from build123d import *

# Parameters (mm, degrees)
EXTRUDE_2_DEPTH     = 1.8
SKETCH_2_R          = 2
CUT_EXTRUDE_3_DEPTH = 1.8


with BuildPart() as part:
    # 草圖1 → 填料-伸長2 (new body)
    with BuildSketch(Plane.XY):
        Polygon((-40.127945462, -52.376209375), (59.872054538, -52.376209375), (82.372054538, -13.405066204), (65.051546462, -3.405066204), (42.551546462, -42.376209375), (-22.807437387, -42.376209375), (-45.307437387, -3.405066204), (-62.627945462, -13.405066204), align=None)
    extrude(amount=EXTRUDE_2_DEPTH)

    # 草圖2 → 除料-伸長3 (cut)
    with BuildSketch(Plane.XY.offset(1.8)):
        with Locations((-48.967691424, -17.065320242)):
            Circle(SKETCH_2_R)
        with Locations((68.7118005, -17.065320242)):
            Circle(SKETCH_2_R)
        with Locations((-43.967691424, -25.72557428)):
            Circle(SKETCH_2_R)
        with Locations((63.7118005, -25.72557428)):
            Circle(SKETCH_2_R)
        with Locations((-15.127945462, -47.376209375)):
            Circle(SKETCH_2_R)
        with Locations((34.872054538, -47.376209375)):
            Circle(SKETCH_2_R)
    extrude(amount=-CUT_EXTRUDE_3_DEPTH, mode=Mode.SUBTRACT)


solid = part.part
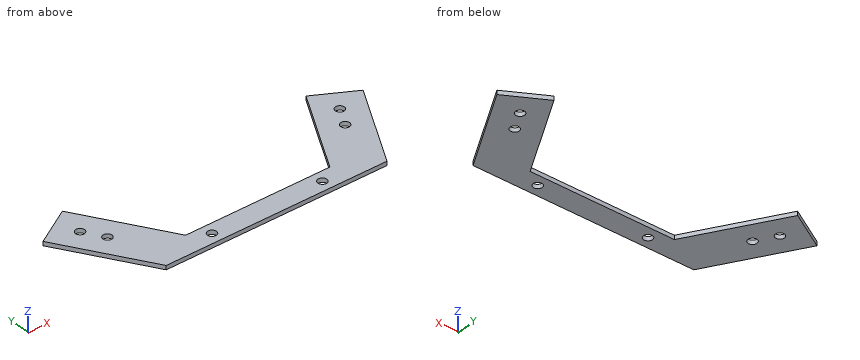
Design review of the part built by this model. Coordinates are the model's own, in mm. Round coordinates to 2 decimals unless told otherwise and drop trailing zeros. Write each loop counter-clockwise with the first axis right and the second up, starting at its lowest first coordinate (ties: lowest second). Pieces come first, ordered by that corner, then holes. Notation, with made-up numbers: (-4.5, 24) - (17.5, 24) arc R21 cw to (17.5, 54) - close; hole circle Ø8 at (60, -15.5). An arc over 180 degrees is marked (long way). Use a Markdown table: item, result. Add a question column.
1. We need section C-C (z = 1). State the section outline as (x, y) points, then the cut area to 3 significant figures.
2. Wall thickness on probe 1 along Y at (x, z) = (-15, 0.8); probe 2 along X at (y, z) = (-26.5, 1.1); probe 3 along X at (y, z) = (-47.5, 0.35): over which ranges is each line inside the solid? List them lowest first.
3. We need section D-D (x = 7.5). State the section outline as (y, z) points, then the cut area to 3 significant figures.
4. We need section A-A (y = -6.5). State the section outline as (x, z) points.
5. Clearance check with a flat-ended pin moving along its axis: pin 1 (0.5 mm diameter, centred on x = 21.5, z = 1, fed in from +Y). State where the tip first meets the part, or that it passes through.
6. We need section B-B (x = 68). State the section outline as (y, z) points, then the cut area to 3 significant figures.
Output:
| question | item | result |
|---|---|---|
| 1 | outline | (-62.63, -13.41) - (-40.13, -52.38) - (59.87, -52.38) - (82.37, -13.41) - (65.05, -3.41) - (42.55, -42.38) - (-22.81, -42.38) - (-45.31, -3.41) - close; hole circle Ø4 at (-48.97, -17.07); hole circle Ø4 at (-43.97, -25.73); hole circle Ø4 at (-15.13, -47.38); hole circle Ø4 at (34.87, -47.38); hole circle Ø4 at (63.71, -25.73); hole circle Ø4 at (68.71, -17.07) |
| 1 | area | 2,550 mm2 |
| 2 | probe 1 | y = -52.38 to -49.37, -45.38 to -42.38 |
| 2 | probe 2 | x = -55.07 to -45.81, -42.12 to -31.97, 51.72 to 61.87, 65.56 to 74.81 |
| 2 | probe 3 | x = -42.94 to -17.12, -13.13 to 32.88, 36.87 to 62.69 |
| 3 | outline | (-52.38, 0) - (-42.38, 0) - (-42.38, 1.8) - (-52.38, 1.8) - close |
| 3 | area | 18.0 mm2 |
| 4 | outline | (-50.67, 0) - (-43.52, 0) - (-43.52, 1.8) - (-50.67, 1.8) - close; (63.26, 0) - (70.41, 0) - (70.41, 1.8) - (63.26, 1.8) - close |
| 5 | pin 1 | stops at y = -42.38 |
| 6 | outline | (-38.3, 0) - (-18.93, 0) - (-18.93, 1.8) - (-38.3, 1.8) - close; (-15.2, 0) - (-5.11, 0) - (-5.11, 1.8) - (-15.2, 1.8) - close |
| 6 | area | 53.0 mm2 |
